Model file for the job. Use its own axes, mm. A direction names the side the tool comes from. Round coordinates to 2 decimals unless told otherwise and drop trailing zeros. Loops run counter-clockwise (first coordinate to the right, second up) from the corner with the lowest first, then second, coordinate; pieces in that order, holes last. Notation, with made-up numbers: M -27,20.25 L 32,20.25 A28 ccw 32,45.25 Z; hole C 26.5,83.25 d10. An arc over 180 degrees is marked long. Use a Markdown table: item, result. Add a question column.
Item 1: Tool access for faces 4 (the flat face through (65, 26, 93.175)), 5 (the cylindrical face through (98.895, 25.22, 121.345)), 6 (the flat face through (1.57, 4.93, 106.21)): list every direction of +Z, -Z, +X, -X, +Y, -Y with a clear straight run to the whole face (end or side of a thin tool).
Item 2: Wall check: L1, parallel to X at y = 10, z = 91 (3 decimals); L2, parallel to Z at x = 48.5, y = 5.5 (3 decimals); L3, parallel to Z at x = 16.5, y = 28 (3 decimals). Give the ranges that are in metal, low to high. Write a range as from..to.
Item 3: Saw through at C-C on y = 25. Write the cut outline in (x, z) (3 decimals).
Item 4: Saw through at B-B on x = 49.5. Write the cut outline in (y, z) (3 decimals), then the cut area to 3 significant figures.
Item 5: Saw through at A-A on z = 58. Write the cut outline in (x, y) (3 decimals), then the cut area to 4 significant figures.
Item 6: Pin check, flat tips, straight feed: P1, Ø2.5, axis at x = -1.5, y = 60, coming from the +Z side; P2, Ø1.5, axis at y = 7.5, z = 71, coming from the +X side; P3, Ø1.6, axis at x = 133, y = -13, coming from the -Z side; P4, Ø1.5, axis at y = -10, z = 43.5, coming from the -X side. Stop position of each tip, or through.
Item 7: Saw through at D-D on y = -7. Write the cut outline in (x, z) (3 decimals).
Item 8: Two-plate mould, pull along Z, no slides. Class faces 1 (the flat face through (1.57, 44.93, 106.49)), 2 (the flat face through (66, 80, 2)), 3 (the flat face through (3.175, 24, 48)): +Z half, -Z half, draft (parallel to the pull), parting line (faces both ways), or undercut.
```python
from build123d import *

# Parameters (mm, degrees)
BOSS_EXTRUDE1_DEPTH = 3.175
SKETCH3_W           = 3.175
SKETCH3_H           = 110
BOSS_EXTRUDE2_DEPTH = 90
BOSS_EXTRUDE3_DEPTH = 3.175
BOSS_EXTRUDE4_DEPTH = 3.175
BOSS_EXTRUDE5_START = -3.175
BOSS_EXTRUDE5_DEPTH = 3.175
SKETCH7_R           = 5
BOSS_EXTRUDE6_DEPTH = 128.475
SKETCH8_R           = 10
BOSS_EXTRUDE7_DEPTH = 5.3
SKETCH10_R          = 2.65


with BuildPart() as part:
    # Sketch2 → Boss-Extrude1 (new body)
    with BuildSketch(Plane.XY):
        Polygon((0, 50), (-3.175, 50), (-3.175, 80), (134.825, 80), (134.825, 50), (131.65, 50), (131.65, 0), (134.825, 0), (134.825, -30), (-3.175, -30), (-3.175, 0), (0, 0), align=None)
    extrude(amount=BOSS_EXTRUDE1_DEPTH)

    # Sketch3 → Boss-Extrude2 (add)
    with BuildSketch(Plane.XY.offset(3.175)):
        with Locations((1.5875, 25)):
            Rectangle(SKETCH3_W, SKETCH3_H)
        with Locations((130.0625, 25)):
            Rectangle(SKETCH3_W, SKETCH3_H)
    extrude(amount=BOSS_EXTRUDE2_DEPTH)

    # Sketch4 → Boss-Extrude3 (add)
    with BuildSketch(Plane.XY.offset(93.175)):
        Polygon((131.65, 50), (134.825, 50), (134.825, 80), (-3.175, 80), (-3.175, 50), (-1.5875, 50), (0, 50), (0, 0), (-3.175, 0), (-3.175, -30), (134.825, -30), (134.825, 0), (131.65, 0), align=None)
    extrude(amount=BOSS_EXTRUDE3_DEPTH)

    # Sketch5 → Boss-Extrude4 (add)
    with BuildSketch(Plane.ZY):
        with BuildLine():
            Line((96.35, 50), (96.35, 0))
            Line((96.35, 0), (116.35, 10))
            ThreePointArc((116.35, 10), (131.35, 25), (116.35, 40))
            Line((116.35, 40), (96.35, 50))
        make_face()
    extrude(amount=-BOSS_EXTRUDE4_DEPTH)

    # Sketch6 → Boss-Extrude5 (add)
    with BuildSketch(Plane(origin=(131.65, 0, 0), x_dir=(0, 0, -1), z_dir=(1, 0, 0)).offset(BOSS_EXTRUDE5_START)):
        with BuildLine():
            Line((-96.35, 0), (-116.35, 10))
            ThreePointArc((-116.35, 10), (-131.35, 25), (-116.35, 40))
            Line((-116.35, 40), (-96.35, 50))
            Line((-96.35, 50), (-96.35, 0))
        make_face()
    extrude(amount=BOSS_EXTRUDE5_DEPTH)

    # Sketch7 → Boss-Extrude6 (add)
    with BuildSketch(Plane(origin=(131.65, 0, 0), x_dir=(0, 0, -1), z_dir=(1, 0, 0))):
        with Locations((-116.35, 25)):
            Circle(SKETCH7_R)
    extrude(amount=-BOSS_EXTRUDE6_DEPTH)

    # Sketch8 → Boss-Extrude7 (add)
    with BuildSketch(Plane.ZY.offset(-68.475)):
        with Locations((116.35, 25)):
            Circle(SKETCH8_R)
    extrude(amount=BOSS_EXTRUDE7_DEPTH)

    # Sketch10 → Cut-Revolve1 (revolve, cut)
    with BuildSketch(Plane(origin=(0, 25, 0), x_dir=(1, 0, 0), z_dir=(0, 1, 0)), mode=Mode.PRIVATE) as cut_revolve1_sk:
        with Locations((65.825, -106.35)):
            Circle(SKETCH10_R)
    revolve(cut_revolve1_sk.sketch.rotate(Axis((63.175, 25, 116.35), (-1, 0, 0)), 180), axis=Axis((63.175, 25, 116.35), (-1, 0, 0)), mode=Mode.SUBTRACT)


solid = part.part
```
Entries:
| question | item | result |
|---|---|---|
| 1 | face 4 | +Y, -Y |
| 1 | face 5 | none |
| 1 | face 6 | +Z, +X, -X, -Y |
| 2 | L1 | 0..3.175, 128.475..131.65 |
| 2 | L2 | 0..3.175, 93.175..96.35 |
| 2 | L3 | 0..3.175, 93.175..96.35, 112.35..120.35 |
| 3 | outline | M 0,0 L 131.65,0 L 131.65,131.35 L 128.475,131.35 L 128.475,121.35 L 68.475,121.35 L 68.475,126.35 A2.65 cw 63.175,126.35 L 63.175,121.35 L 3.175,121.35 L 3.175,131.35 L 0,131.35 Z; hole M 3.175,3.175 L 128.475,3.175 L 128.475,93.175 L 3.175,93.175 Z; hole M 3.175,96.35 L 128.475,96.35 L 128.475,111.35 L 68.475,111.35 L 68.475,106.35 A2.65 ccw 63.175,106.35 L 63.175,111.35 L 3.175,111.35 Z |
| 4 | outline | M -30,0 L 80,0 L 80,3.175 L -30,3.175 Z; M -30,93.175 L 80,93.175 L 80,96.35 L -30,96.35 Z; C 25,116.35 d10 |
| 4 | area | 777 mm2 |
| 5 | outline | M 0,-30 L 3.175,-30 L 3.175,80 L 0,80 Z; M 128.475,-30 L 131.65,-30 L 131.65,80 L 128.475,80 Z |
| 5 | area | 698.5 mm2 |
| 6 | P1 | z = 96.35 |
| 6 | P2 | x = 131.65 |
| 6 | P3 | z = 0 |
| 6 | P4 | x = 0 |
| 7 | outline | M -3.175,0 L 134.825,0 L 134.825,3.175 L 131.65,3.175 L 131.65,93.175 L 134.825,93.175 L 134.825,96.35 L -3.175,96.35 L -3.175,93.175 L 0,93.175 L 0,3.175 L -3.175,3.175 Z; hole M 3.175,3.175 L 128.475,3.175 L 128.475,93.175 L 3.175,93.175 Z |
| 8 | face 1 | +Z half |
| 8 | face 2 | draft |
| 8 | face 3 | undercut |
